```python
from build123d import *

# Parameters (mm, degrees)
F0_W      = 55.562247
F0_H      = 56.532964
F1_DEPTH  = 55.88
F3_DEPTH  = 143.764
F5_DEPTH  = 45.466
F7_DEPTH  = 94.742
F9_DEPTH  = 254
F10_W     = 102.854468
F10_H     = 33.626976
F11_DEPTH = 128.524
F12_W     = 127.998766
F12_H     = 88.431828
F13_DEPTH = 11.43


with BuildPart() as f1:
    # F0 (on Front) → F1 (new body)
    with BuildSketch(Plane.XZ):
        with Locations((-1.708673, 28.266482)):
            Rectangle(F0_W, F0_H)
    extrude(amount=F1_DEPTH)

    # F2 (on Front) → F3 (cut)
    with BuildSketch(Plane.XZ):
        Polygon((0, 58.050822), (27.564345, 0), (27.564345, 58.050822), align=None)
    extrude(amount=F3_DEPTH, mode=Mode.SUBTRACT)

    # F4 (on Right) → F5 (cut, symmetric)
    with BuildSketch(Plane.YZ):
        Polygon((-62.023856, 67.624263), (-61.119623, 0), (-15.732997, 67.624263), align=None)
    extrude(amount=F5_DEPTH, both=True, mode=Mode.SUBTRACT)

    # F6 (on face) → F7 (cut)
    with BuildSketch(Plane(origin=(-29.489797, 0, 0), x_dir=(0, -1, 0), z_dir=(-1, 0, 0))):
        Polygon((0, 0), (23.177022, 56.532964), (0, 56.532964), align=None)
    extrude(amount=-F7_DEPTH, mode=Mode.SUBTRACT)

    # F8 (on Front) → F9 (cut)
    with BuildSketch(Plane.XZ):
        Polygon((-39.340276, 63.730873), (-28.191272, 0), (0, 63.730873), align=None)
    extrude(amount=F9_DEPTH, mode=Mode.SUBTRACT)

    # F10 (on Front) → F11 (cut)
    with BuildSketch(Plane.XZ):
        with Locations((-6.703854, -8.482341)):
            Rectangle(F10_W, F10_H)
    extrude(amount=F11_DEPTH, mode=Mode.SUBTRACT)

    # F12 (on Top) → F13 (cut)
    with BuildSketch(Plane.XY):
        with Locations((12.506837, -16.333792)):
            Rectangle(F12_W, F12_H)
    extrude(amount=F13_DEPTH, mode=Mode.SUBTRACT)


solid = f1.part
```
Read the model definition and answer for the solid it produces. Units are mm, in the model's axes. Coordinates: 2 decimals unless noted, no trailing zeros. Order: outer loops, then holes, each group sorted by start corner. A loop starts at its lowest first (then second) coordinate and runs counter-clockwise, first axis right, second up. Notation, with made-up numbers: (27.25, 39) - (43.25, 39) arc R23 ccw to (43.25, 57) - close; hole circle Ø7 at (48.5, 15). An arc over 180 degrees is marked (long way). Answer as a JSON object with one key per item and string values. Group by question number.
Item 1: Consider probe 1 along X at (y, z) = (-30.5, 35); probe 2 along Z at (x, y) = (-13, -50.5); probe 3 along Y at (x, z) = (8.5, 33.5). Determine where each line is inside the solid, lowest interval first. Write a range as from..to.
Item 2: Flat-ended cylindrical pins translate along their axes: P1, Ø10, axis at x = -11, y = -36, coming from the +Z side; P2, Ø5, axis at x = -2, z = 22.5, coming from the +Y side; P3, Ø10, axis at y = -20.5, z = 51, coming from the +X side. Find the tip coordinate at first contact, or state that the pin passes through.
Item 3: Section A-A (y = -40.5) is taken. Give the vertices of the cut face in (x, z), plus the area to 3 significant figures.
Item 4: Section B-B (x = -19) is taken. Give the vertices of the cut face in (y, z), plus the area to 3 significant figures.
Results are:
{
 "1": {"probe 1": "x = -12.71..10.95", "probe 2": "z = 11.43..15.82", "probe 3": "y = -38.64..-13.73"},
 "2": {"P1": "stops at z = 44.05", "P2": "stops at y = -8.2", "P3": "stops at x = 5.72"},
 "3": {"outline": "(-23.14, 11.43) - (22.14, 11.43) - (12.98, 30.72) - (-14.6, 30.72) - close", "area": "703 mm^2"},
 "4": {"outline": "(-53.45, 11.43) - (-4.69, 11.43) - (-8.52, 20.78) - (-47.17, 20.78) - close", "area": "409 mm^2"}
}
